For this review, use the dimensioned drawing (mm, ordinates from the lowest corner) and the shaded views. Round coordinates to 2 decimals unless told otherwise and drop trailing zeros. Loops run counter-clockwise (first coordinate to the right, second up) from the corner with the lowest first, then second, coordinate; pieces in that order, holes last. Notation, with made-up numbers: M -22,48.25 L 7,48.25 A20 cw 7,52.25 Z; hole C -20.75,29 d10. An arc over 180 degrees is marked long. One line per item, written item: value. Start each with the question number.
Item 1: We need section D-D (x = 48.5). Write out the cut boundary in (y, z), then the cut area to 3 significant figures.
Item 2: We need section B-B (y = 12.7). Write out the cut boundary in (x, z), then the cut area to 3 significant figures.
Item 3: We need section C-C (z = 1.75). Write out the cut boundary in (x, y), then the cut area to 3 significant figures.
Item 4: For line 1 along Y through (x, z) = (9.5, 2.65); line 2 along Y through (x, z) = (35, 2); line 3 along X through (y, z) = (97.5, 5.1), list the stretches that pass through material, from the lowest coordinate up.
Item 5: We need section A-A (x = 9.5). Write out the cut boundary in (y, z), then the cut area to 3 significant figures.
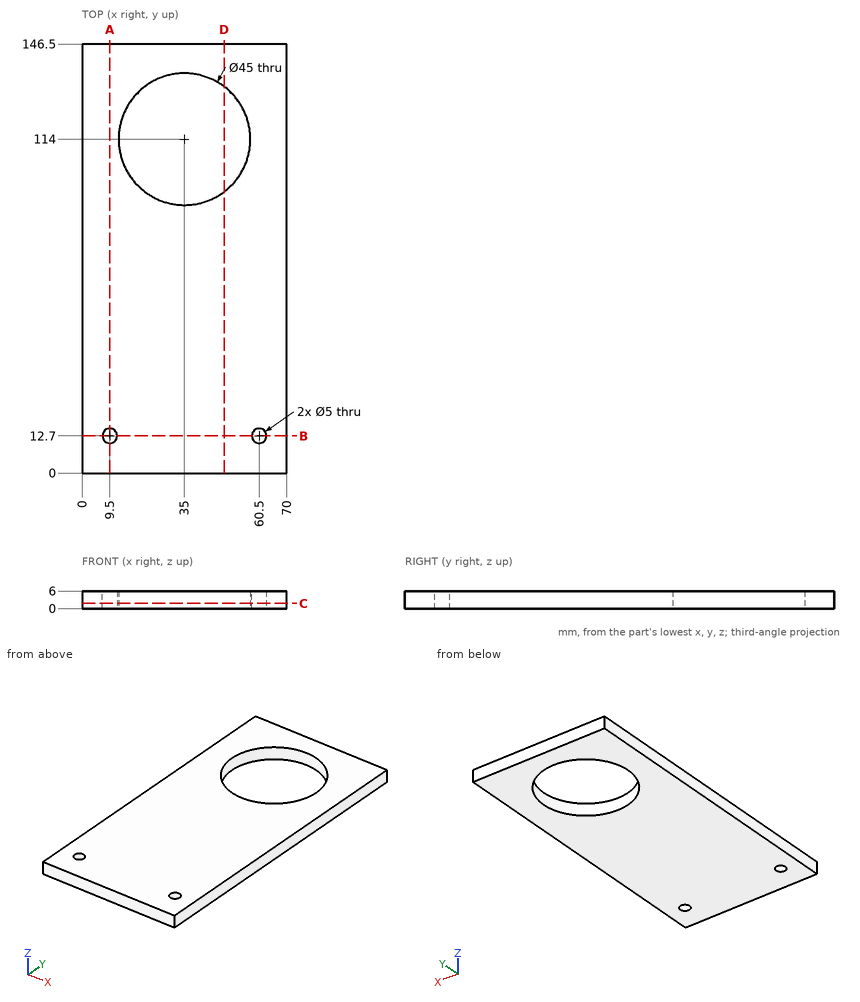
A:
1. outline: M 0,0 L 96,0 L 96,6 L 0,6 Z; M 132,0 L 146.5,0 L 146.5,6 L 132,6 Z
1. area: 663 mm2
2. outline: M 0,0 L 7,0 L 7,6 L 0,6 Z; M 12,0 L 58,0 L 58,6 L 12,6 Z; M 63,0 L 70,0 L 70,6 L 63,6 Z
2. area: 360 mm2
3. outline: M 0,0 L 70,0 L 70,146.5 L 0,146.5 Z; hole C 9.5,12.7 d5; hole C 35,114 d45; hole C 60.5,12.7 d5
3. area: 8,630 mm2
4. line 1: 0 to 10.2, 15.2 to 146.5
4. line 2: 0 to 91.5, 136.5 to 146.5
4. line 3: 0 to 19.7, 50.3 to 70
5. outline: M 0,0 L 10.2,0 L 10.2,6 L 0,6 Z; M 15.2,0 L 146.5,0 L 146.5,6 L 15.2,6 Z
5. area: 849 mm2
